from build123d import *

# Parameters (mm, degrees)
BOSS_EXTRUDE1_DEPTH      = 86.36
BOSS_EXTRUDE1_DEPTH_BACK = 86.36
SKETCH3_W                = 172.72
SKETCH3_H                = 0.4064
SKETCH4_R                = 7.800000021
CUT_EXTRUDE1_DEPTH       = 123.132159405
SKETCH6_R                = 1.524
SKETCH6_R_2              = 1
CUT_EXTRUDE2_DEPTH       = 123.132159405


with BuildPart() as part:
    # Sketch3 → Boss-Extrude1 (new, two sides: drawn at the far end of the back side and taken through both)
    with BuildSketch(Plane.XY.offset(-BOSS_EXTRUDE1_DEPTH_BACK)):
        Rectangle(SKETCH3_W, SKETCH3_H)
    extrude(amount=BOSS_EXTRUDE1_DEPTH + BOSS_EXTRUDE1_DEPTH_BACK)

    # Sketch4 → Cut-Extrude1 (cut, through all)
    with BuildSketch(Plane(origin=(0, 0.2032, 0), x_dir=(1, 0, 0), z_dir=(0, 1, 0))):
        with Locations(Location((40.04, -66.04, 0), (0, 0, 270))):
            Circle(SKETCH4_R)
        with Locations(Location((66.04, -66.04, 0), (0, 0, 270))):
            Circle(SKETCH4_R)
    extrude(amount=-CUT_EXTRUDE1_DEPTH, mode=Mode.SUBTRACT)

    # Sketch6 → Cut-Extrude2 (cut, through all)
    with BuildSketch(Plane.XZ.offset(0.2032)):
        with Locations(Location((-20.32, 20.32, 0), (0, 0, 270))):
            Circle(SKETCH6_R)
        with Locations(Location((68.58, 20.32, 0), (0, 0, 270))):
            Circle(SKETCH6_R)
        with Locations(Location((68.58, -68.58, 0), (0, 0, 270))):
            Circle(SKETCH6_R)
        with Locations(Location((-20.32, -68.58, 0), (0, 0, 270))):
            Circle(SKETCH6_R)
        with Locations(Location((-20.32, 33.02, 0), (0, 0, 270))):
            Circle(SKETCH6_R)
        with Locations(Location((-20.32, 63.52032, 0), (0, 0, 270))):
            Circle(SKETCH6_R)
        with Locations(Location((10.18032, 63.52032, 0), (0, 0, 270))):
            Circle(SKETCH6_R)
        with Locations(Location((10.18032, 33.02, 0), (0, 0, 270))):
            Circle(SKETCH6_R)
        with Locations(Location((-45.72, 45.74032153, 0), (0, 0, 270))):
            Circle(SKETCH6_R_2)
        with Locations(Location((-30.48, 63.52032, 0), (0, 0, 270))):
            Circle(SKETCH6_R_2)
    extrude(amount=-CUT_EXTRUDE2_DEPTH, mode=Mode.SUBTRACT)


solid = part.part
Input: part model. Units: mm. Frame: model coordinates. Give positions to 0.01 mm unless a question says otherwise; leave off trailing zeros. Write each loop counter-clockwise with the first axis right and the second up, starting at its lowest first coordinate (ties: lowest second). Pieces come first, ordered by that corner, then holes.
Q1. Pull-direction query (Z, two-part tool) for faces 1 (the face through (72.62, 0, 70.23)), 2 (the face through (-1, 0.203, -1)); classes: pulls with the +Z half, pulls with the -Z half, needs draft (parallel to the pull), parting line crosses it, or undercut.
Q2. Material intervals for probe 1 along X at (y, z) = (0.15, 66); probe 2 along X at (y, z) = (0, 33.02); probe 3 along Z at (x, y) = (39.5, 0.1), sorted ascending.
Q3. Section A-A, the plane x = 42.5. Output: boundary loops of the cut face in (y, z).
Q4. First-contact query: P1, Ø3.5, axis at x = 68.58, z = -68.58, coming from the +Y side. Flat tip, straight axial feed; report the tip coordinate or a pass-through.
Filled in:
1. face 1: undercut
1. face 2: needs draft
2. probe 1: x = -86.36 to 32.24, 47.84 to 58.24, 73.84 to 86.36
2. probe 2: x = -86.36 to -21.84, -18.8 to 8.66, 11.7 to 86.36
2. probe 3: z = -86.36 to 58.26, 73.82 to 86.36
3. outline: (-0.2, -86.36) - (0.2, -86.36) - (0.2, 58.64) - (-0.2, 58.64) - close; (-0.2, 73.44) - (0.2, 73.44) - (0.2, 86.36) - (-0.2, 86.36) - close
4. P1: stops at y = 0.2
